from build123d import *

# Parameters (mm, degrees)
MAIN_BODY_DEPTH    = 10.5
RIB1_REACH         = 45.385
SKETCH2_WALL_W     = 117.37050971
SKETCH2_WALL_H     = 3
SKETCH3_R          = 7.5
SHAFT_DEPTH        = 8
CUT_EXTRUDE1_START = -5.3
CUT_EXTRUDE1_DEPTH = 5.3
CUT_EXTRUDE2_START = -13.3
SKETCH6_R          = 7.5
CUT_EXTRUDE2_DEPTH = 13.3
SKETCH7_R          = 1.95
CUT_EXTRUDE3_DEPTH = 42.082112896


with BuildPart() as part:
    # Sketch1 → Main Body (new, symmetric)
    with BuildSketch(Plane.XY):
        with BuildLine():
            Line((-7.5, 0), (-7.5, -29))
            Line((-7.5, -29), (24.5, -29))
            Line((24.5, -29), (24.5, -23))
            Line((24.5, -23), (7.5, -23))
            Line((7.5, -23), (7.5, 0))
            ThreePointArc((7.5, 0), (0, 7.5), (-7.5, 0))
        make_face()
    main_body = extrude(amount=MAIN_BODY_DEPTH, both=True)

    # Sketch2 wall → Rib1 (add, up to next)
    with BuildSketch(Plane(origin=(16, -11.5, 10.5), x_dir=(0.594391061084, -0.804176141466, 0), z_dir=(0.804176141466, 0.594391061084, 0)), mode=Mode.PRIVATE) as rib1_sk1:
        with Locations((0, 1.5)):
            Rectangle(SKETCH2_WALL_W, SKETCH2_WALL_H)
    rib1_tool1 = extrude(rib1_sk1.sketch, amount=-RIB1_REACH, mode=Mode.PRIVATE) - part.part
    rib1 = rib1_tool1.solids().sort_by_distance((16, -11.5, 10.5))[0]
    add(rib1)

    # Sketch3 → Shaft (add)
    with BuildSketch(Plane.XY.offset(-10.5)):
        Circle(SKETCH3_R)
    extrude(amount=-SHAFT_DEPTH)

    # Mirror2: Main Body, Rib1 across plane
    add(main_body.mirror(Plane(origin=(0, 0, 0), x_dir=(0, 0, 1), z_dir=(1, 0, 0))))
    add(rib1.mirror(Plane(origin=(0, 0, 0), x_dir=(0, 0, 1), z_dir=(1, 0, 0))))

    # Sketch5 → Cut-Extrude1 (cut)
    with BuildSketch(Plane(origin=(0, 0, -10.5), x_dir=(-1, 0, 0), z_dir=(0, 0, -1)).offset(CUT_EXTRUDE1_START)):
        with BuildLine():
            Line((-7.5, 0), (-7.5, -23))
            Line((-7.5, -23), (-24.5, -23))
            Line((-24.5, -23), (-24.5, -29))
            Line((-24.5, -29), (24.5, -29))
            Line((24.5, -29), (24.5, -23))
            Line((24.5, -23), (7.5, -23))
            Line((7.5, -23), (7.5, 0))
            ThreePointArc((7.5, 0), (0, -7.5), (-7.5, 0))
        make_face()
    extrude(amount=CUT_EXTRUDE1_DEPTH, mode=Mode.SUBTRACT)

    # Sketch6 → Cut-Extrude2 (cut)
    with BuildSketch(Plane(origin=(0, 0, -18.5), x_dir=(-1, 0, 0), z_dir=(0, 0, -1)).offset(CUT_EXTRUDE2_START)):
        Circle(SKETCH6_R)
    extrude(amount=CUT_EXTRUDE2_DEPTH, mode=Mode.SUBTRACT)

    # Sketch7 → Cut-Extrude3 (cut, through all)
    with BuildSketch(Plane.XY.offset(10.5)):
        Circle(SKETCH7_R)
    extrude(amount=-CUT_EXTRUDE3_DEPTH, mode=Mode.SUBTRACT)


solid = part.part
Work out the finished part from the listing and answer in its coordinate system (mm). A direction names the side the tool comes from. Give positions to 0.01 mm unless a question says otherwise; leave off trailing zeros. Order: outer loops, then holes, each group sorted by start corner. A loop starts at its lowest first (then second) coordinate and runs counter-clockwise, first axis right, second up. Notation, with made-up numbers: (-20.75, 28.25) -> (25.25, 28.25) arc R17 ccw to (25.25, 38.25) -> close; hole circle Ø10 at (-20.5, 9). An arc over 180 degrees is marked (long way). One line per item, written item: value.
Item 1: Find section D-D, the plane x = 17. Give the vertices of the cut face in (y, z), plus the area to 3 significant figures.
Answer sheet:
outline: (-29, -5.2) -> (-23, -5.2) -> (-23, 7.5) -> (-12.85, 7.5) -> (-12.85, 10.5) -> (-29, 10.5) -> close
area: 125 mm²
Item 2: Find section A-A, the plane x = 0. Give the vertices of the cut face in (y, z).
Answer sheet:
outline: (-29, -5.2) -> (-1.95, -5.2) -> (-1.95, 10.5) -> (-29, 10.5) -> close; (1.95, -5.2) -> (7.5, -5.2) -> (7.5, 10.5) -> (1.95, 10.5) -> close
Item 3: Flat-ended cylindrical pins translate along their axes: P1, Ø6, axis at y = -16.5, z = -3, coming from the +X side; P2, Ø5, axis at x = 13.5, y = -12.5, coming from the -Z side; P3, Ø4, axis at y = -14.5, z = -0.5, coming from the -X side; P4, Ø10, axis at x = 15, y = 3.5, coming from the -Z side. Find the tip coordinate at first contact, or state that the pin passes through.
Answer sheet:
P1: x = 7.5
P2: z = 7.5
P3: x = -7.5
P4: through
Item 4: Find section B-B, the plane z = 1. Give the vertices of the cut face in (x, y).
Answer sheet:
outline: (-24.5, -29) -> (24.5, -29) -> (24.5, -23) -> (7.5, -23) -> (7.5, 0) arc R7.5 ccw to (-7.5, 0) -> (-7.5, -23) -> (-24.5, -23) -> close; hole circle Ø3.9 at (0, 0)
Item 5: A tool of negligible diameter and unlimited length cuts with its end or side. For faces 1 (the flat face through (0, -15, -5.2)), 2 (the flat face through (-7.5, -11, 1)), 3 (the flat face through (13, -14, 7.5)), from which of +Z, -Z, +X, -X, +Y, -Y can it reach the whole face along a straight path? Write none if from no direction.
Answer sheet:
face 1: -Z, +X, -X, +Y, -Y
face 2: -Z, -X, +Y
face 3: -Z, +X, +Y
Item 6: Straight lines are drawn through the part: probe 1 along Y at (x, z) = (0, 3); probe 2 along X at (y, z) = (-22, -4); probe 3 along Z at (x, y) = (12, -8). For each, find the intervals that lie inside material, in ascending order.
Answer sheet:
probe 1: -29 to -1.95, 1.95 to 7.5
probe 2: -7.5 to 7.5
probe 3: 7.5 to 10.5
Item 7: Determine the mould class of faces 4 (the flat face through (-16, -23, 1)), 5 (the cylindrical face through (-1.437, 1.318, 2.76)), 6 (the flat face through (-1, -18, 10.5)), 7 (the flat face through (0, -29, 3)) for opening direction Y: released by +Y, released by -Y, zero draft, split by the parting line, or undercut.
Answer sheet:
face 4: released by +Y
face 5: undercut
face 6: zero draft
face 7: released by -Y
Item 8: Find section C-C, the plane z = 9. Give the vertices of the cut face in (x, y), plus the area to 3 significant figures.
Answer sheet:
outline: (-24.5, -29) -> (24.5, -29) -> (24.5, -23) -> (7.5, 0) arc R7.5 ccw to (-7.5, 0) -> (-24.5, -23) -> close; hole circle Ø3.9 at (0, 0)
area: 1,110 mm²
